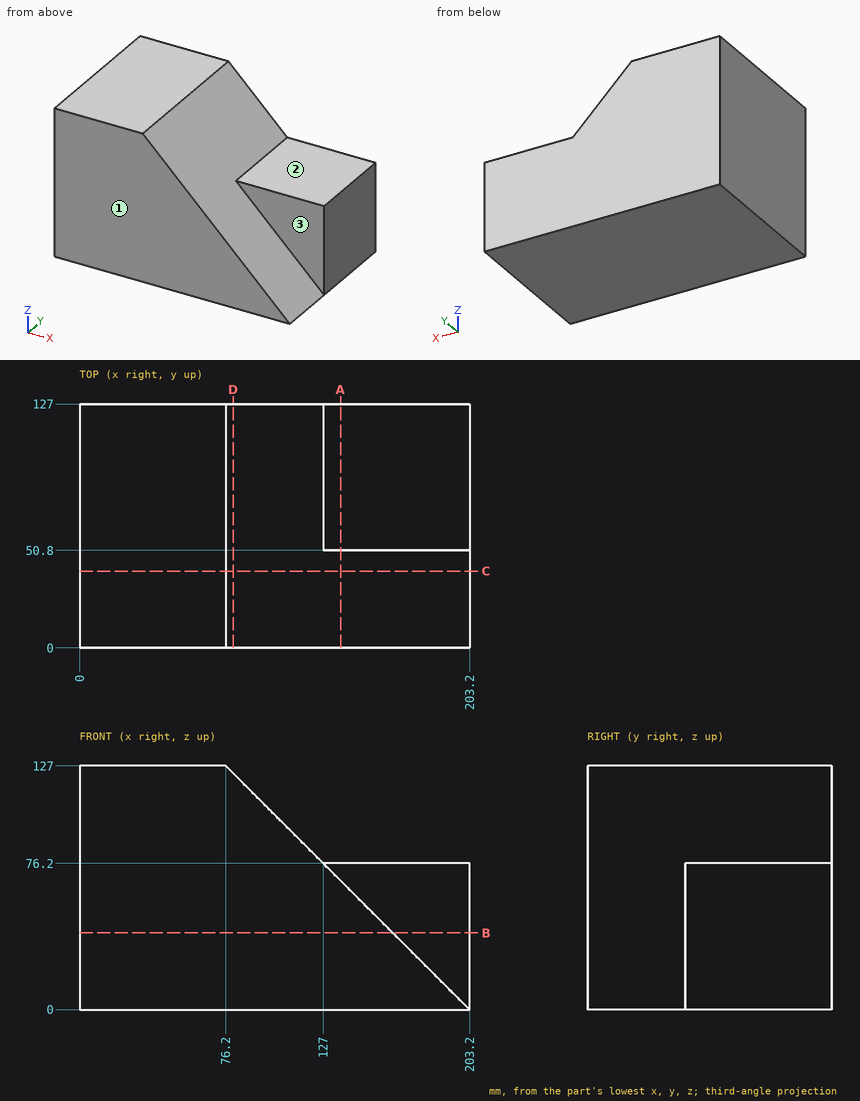
Geometry check sheet. Reference: drawing and pictorial views, mm from the part's lowest x, y, z. A direction names the side the tool comes from. Round coordinates to 2 decimals unless told otherwise and drop trailing zeros. Loops run counter-clockwise (first coordinate to the right, second up) from the corner with the lowest first, then second, coordinate; pieces in that order, holes last. Notation, with made-up numbers: (53, 86) - (73, 86) arc R32 cw to (73, 124) - close; hole circle Ø9 at (-39, 25.25). An arc over 180 degrees is marked (long way). Answer in a Markdown table with one row per item. Add a question column.
Q1. Gauge pin test, flat ends, axial feed: pin 1 (1 mm diameter, centred on y = 60.5, z = 98.5, fed in from +X); pin 2 (3 mm diameter, centred on x = 119, y = 14, fed in from +Z); pin 3 (8 mm diameter, centred on y = 80.5, z = 94.5, fed in from +X). Record the tip position at first contact, or that the pin passes through.
Q2. Material ranges on line 1 (Z direction, x = 194.5, y = 51.5); line 2 (X direction, y = 65.5, z = 98.5); line 3 (Z direction, x = 166.5, y = 9), recorded low to high.
Q3. Section check D-D on x = 80. Enter the section's corners in (y, z).
Q4. Tool access check on the marked faces 1, 2 and 3. Record the directions out of +Z, -Z, +X, -X, +Y, -Y that give a thin tool (end or side, any length) a straight path to the whole face; none if there is none.
Q5. Section check B-B on z = 40. Enter the section's corners in (x, y).
Q6. Section check A-A on x = 136. Enter the section's corners in (y, z), plus the area to 3 significant figures.
Q7. Section check C-C on y = 40. Enter the section's corners in (x, z), plus the area to 3 significant figures.
Found:
| question | item | result |
|---|---|---|
| 1 | pin 1 | stops at x = 105.2 |
| 1 | pin 2 | stops at z = 85.7 |
| 1 | pin 3 | stops at x = 112.7 |
| 2 | line 1 | z = 0 to 76.2 |
| 2 | line 2 | x = 0 to 104.7 |
| 2 | line 3 | z = 0 to 36.7 |
| 3 | outline | (0, 0) - (127, 0) - (127, 123.2) - (0, 123.2) - close |
| 4 | face 1 | +Z, -Z, +X, -X, -Y |
| 4 | face 2 | +Z, +X, +Y, -Y |
| 4 | face 3 | +Z, +X, -Y |
| 5 | outline | (0, 0) - (163.2, 0) - (163.2, 50.8) - (203.2, 50.8) - (203.2, 127) - (0, 127) - close |
| 6 | outline | (0, 0) - (127, 0) - (127, 76.2) - (50.8, 76.2) - (50.8, 67.2) - (0, 67.2) - close |
| 6 | area | 9,220 mm² |
| 7 | outline | (0, 0) - (203.2, 0) - (76.2, 127) - (0, 127) - close |
| 7 | area | 17,700 mm² |
